from build123d import *

# Parameters (mm, degrees)
F1_DEPTH      = 1524
F2_R          = 6.35
F3_DEPTH      = 22.226
F3_DEPTH_BACK = 22.226


with BuildPart() as f1:
    # F0 (on Front) → F1 (new body)
    with BuildSketch(Plane.XZ):
        Polygon((-22.225, 0), (0, 0), (22.225, 0), (22.225, 53.975), (12.7, 53.975), (12.7, 9.525), (-12.7, 9.525), (-12.7, 53.975), (-22.225, 53.975), align=None)
    extrude(amount=F1_DEPTH)

    # F2 (on Right) → F3 (cut, two sides)
    with BuildSketch(Plane.YZ) as f3_sk:
        with Locations((-38.1, 34.925)):
            Circle(F2_R)
        with Locations((-134.62, 34.925)):
            Circle(F2_R)
        with Locations((-231.14, 34.925)):
            Circle(F2_R)
        with Locations((-327.66, 34.925)):
            Circle(F2_R)
        with Locations((-424.18, 34.925)):
            Circle(F2_R)
        with Locations((-520.7, 34.925)):
            Circle(F2_R)
        with Locations((-617.22, 34.925)):
            Circle(F2_R)
        with Locations((-713.74, 34.925)):
            Circle(F2_R)
        with Locations((-810.26, 34.925)):
            Circle(F2_R)
        with Locations((-906.78, 34.925)):
            Circle(F2_R)
        with Locations((-1003.3, 34.925)):
            Circle(F2_R)
        with Locations((-1099.82, 34.925)):
            Circle(F2_R)
        with Locations((-1196.34, 34.925)):
            Circle(F2_R)
        with Locations((-1292.86, 34.925)):
            Circle(F2_R)
        with Locations((-1389.38, 34.925)):
            Circle(F2_R)
        with Locations((-1485.9, 34.925)):
            Circle(F2_R)
    extrude(amount=F3_DEPTH, mode=Mode.SUBTRACT)
    extrude(f3_sk.sketch, amount=-F3_DEPTH_BACK, mode=Mode.SUBTRACT)


solid = f1.part
Read the model definition and answer for the solid it produces. Units are mm, in the model's axes. A direction names the side the tool comes from. Coordinates: 2 decimals unless noted, no trailing zeros. Write each loop counter-clockwise with the first axis right and the second up, starting at its lowest first coordinate (ties: lowest second). Pieces come first, ordered by that corner, then holes. Notation, with made-up numbers: (49, 79) -> (80, 79) arc R21 ccw to (80, 117) -> close; hole circle Ø9 at (79, 77.5). An arc over 180 degrees is marked (long way). Return JSON: item names as keys, results as strings.
(1) Which of the six approach directions +Z, -Z, +X, -X, +Y, -Y give full straight-line access (tool end or side, diameter ignored) to faces 1 (the flat face through (22.225, -751, 27)), 2 (the flat face through (-12.7, -751, 31))?
Answers below:
{"face 1": "+Z, -Z, +X, +Y, -Y", "face 2": "+Z, +Y, -Y"}
(2) Consider line 1 along X through (y, z) = (-974, 19.5) (3 decimals); line 2 along Z through (x, y) = (18, -1099) (3 decimals); line 3 along Z through (x, y) = (19, -38) (3 decimals). Determine where each line is inside the solid, lowest interval first. Write a range as from..to.
Answers below:
{"line 1": "-22.225..-12.7, 12.7..22.225", "line 2": "0..28.628, 41.222..53.975", "line 3": "0..28.576, 41.274..53.975"}
(3) The part is cut by section B-B on x = -2.5. Give the vertices of the cut face in (y, z) (3 decimals), then the cut area to 3 significant figures.
Answers below:
{"outline": "(-1524, 0) -> (0, 0) -> (0, 9.525) -> (-1524, 9.525) -> close", "area": "14,500 mm^2"}
(4) For a pull along X with two mould halves and no side action, classify faces 3 (the flat face through (0, -751, 0)), 4 (the flat face through (-22.225, -751, 27)), 5 (the flat face through (0, -751, 9.525)) as pulls with the +X half, pulls with the -X half, needs draft (parallel to the pull), parting line crosses it, or undercut.
Answers below:
{"face 3": "needs draft", "face 4": "pulls with the -X half", "face 5": "undercut"}
(5) This flat-tipped pin is pushed along its axis until it touches: P1, Ø8, axis at x = -8, y = -1366, coming from the +Z side (3 decimals). Where does it stop, or does it pass through?
Answers below:
{"P1": "z = 9.525"}
(6) The part is cut by section A-A on y = -1123.5. Give the vertices of the cut face in (x, z) (3 decimals), then the cut area to 3 significant figures.
Answers below:
{"outline": "(-22.225, 0) -> (22.225, 0) -> (22.225, 53.975) -> (12.7, 53.975) -> (12.7, 9.525) -> (-12.7, 9.525) -> (-12.7, 53.975) -> (-22.225, 53.975) -> close", "area": "1,270 mm^2"}
